from build123d import *

# Parameters (mm, degrees)
SKIZZE1_W                                            = 180
SKIZZE1_H                                            = 180
AUFSATZ_LINEAR_AUSTRAGEN1_DEPTH                      = 5
AUFSATZ_LINEAR_AUSTRAGEN2_DEPTH                      = 2
STIRNSENKUNG_F_R_M3_ZYLINDERSCHRAUBE_MIT_D           = 3.6
STIRNSENKUNG_F_R_M3_ZYLINDERSCHRAUBE_MIT_DEPTH       = 9.1
STIRNSENKUNG_F_R_M3_ZYLINDERSCHRAUBE_MIT_CBORE_D     = 6.5
STIRNSENKUNG_F_R_M3_ZYLINDERSCHRAUBE_MIT_CBORE_DEPTH = 3.4
STIRNSENKUNG_F_R_M3_ZYLINDERSCHRAUBE_MIT_TIP         = 1.081549114
VERRUNDUNG1_R                                        = 10
VERRUNDUNG2_R                                        = 2


with BuildPart() as part:
    # Skizze1 → Aufsatz-Linear austragen1 (new body)
    with BuildSketch(Plane(origin=(0, 0, 0), x_dir=(1, 0, 0), z_dir=(0, 1, 0))):
        Rectangle(SKIZZE1_W, SKIZZE1_H)
    extrude(amount=AUFSATZ_LINEAR_AUSTRAGEN1_DEPTH)

    # Skizze2 → Aufsatz-Linear austragen2 (add)
    with BuildSketch(Plane(origin=(0, 5, 0), x_dir=(1, 0, 0), z_dir=(0, 1, 0))):
        with BuildLine():
            Line((78, 85), (-78, 85))
            ThreePointArc((-78, 85), (-85.071067812, 82.071067812), (-88, 75))
            Line((-88, 75), (-88, -75))
            ThreePointArc((-88, -75), (-85.071067812, -82.071067812), (-78, -85))
            Line((-78, -85), (78, -85))
            ThreePointArc((78, -85), (85.071067812, -82.071067812), (88, -75))
            Line((88, -75), (88, 75))
            ThreePointArc((88, 75), (85.071067812, 82.071067812), (78, 85))
        make_face()
    extrude(amount=AUFSATZ_LINEAR_AUSTRAGEN2_DEPTH)

    # Stirnsenkung für M3 Zylinderschraube mit Innensechskant2
    with Locations(Plane(origin=(0, 0, 0), x_dir=(-1, 0, 0), z_dir=(0, -1, 0))):
        with Locations((-83, 80), (83, 80), (83, -80), (-83, -80)):
            CounterBoreHole(STIRNSENKUNG_F_R_M3_ZYLINDERSCHRAUBE_MIT_D / 2, STIRNSENKUNG_F_R_M3_ZYLINDERSCHRAUBE_MIT_CBORE_D / 2, STIRNSENKUNG_F_R_M3_ZYLINDERSCHRAUBE_MIT_CBORE_DEPTH, depth=STIRNSENKUNG_F_R_M3_ZYLINDERSCHRAUBE_MIT_DEPTH)
            with Locations((0, 0, -(STIRNSENKUNG_F_R_M3_ZYLINDERSCHRAUBE_MIT_DEPTH + STIRNSENKUNG_F_R_M3_ZYLINDERSCHRAUBE_MIT_TIP / 2))):  # 118° drill point
                Cone(0, STIRNSENKUNG_F_R_M3_ZYLINDERSCHRAUBE_MIT_D / 2, STIRNSENKUNG_F_R_M3_ZYLINDERSCHRAUBE_MIT_TIP, mode=Mode.SUBTRACT)

    # Verrundung1
    verrundung1_edges = [part.edges().sort_by_distance(p)[0] for p in [
        (90, 2.5, -90),
        (90, 2.5, 90),
        (-90, 2.5, 90),
        (-90, 2.5, -90),
    ]]
    fillet(verrundung1_edges, radius=VERRUNDUNG1_R)

    # Verrundung2
    verrundung2_edges = [part.edges().sort_by_distance(p)[0] for p in [
        (90, 0, 0),
        (0, 0, -90),
        (0, 0, 90),
        (-90, 0, 0),
        (87.071067812, 0, -87.071067812),
        (-87.071067812, 0, -87.071067812),
        (-87.071067812, 0, 87.071067812),
        (87.071067812, 0, 87.071067812),
    ]]
    fillet(verrundung2_edges, radius=VERRUNDUNG2_R)


solid = part.part
Could you check a few things on this model? Use its own coordinates, in mm. A direction names the side the tool comes from. Give positions to 0.01 mm unless a question says otherwise; leave off trailing zeros. Write each loop counter-clockwise with the first axis right and the second up, starting at its lowest first coordinate (ties: lowest second). Pieces come first, ordered by that corner, then holes. Notation, with made-up numbers: (79.25, 34.25) - (105.25, 34.25) arc R18 ccw to (105.25, 64.25) - close; hole circle Ø7 at (-22, -7). An arc over 180 degrees is marked (long way). Use CSV: the item, a comma, the result in double quotes. Start each with the question number.
Item 1: For faces 1 (the face through (-85.15, 5.99, 81.99)), 2 (the face through (-84.4, 3.4, 81.4)), 3 (the face through (84.99, 5.99, 82.15)), 4 (the face through (-84.99, 5.99, -82.15)), which set-ups out of +Z, -Z, +X, -X, +Y, -Y let a thin tool reach every point of the face, with its end or its side?
Item 2: I'm going to push flat-ended pins straight in: pin 1 (4 mm diameter, centred on x = -83, z = 80, fed in from -Y); pin 2 (1 mm diameter, centred on y = 6, z = 16.5, fed in from -X); pin 3 (1.6 mm diameter, centred on x = 9.5, y = 6, fed in from -Z). Where does each tip first touch, or does it pass through?
Item 3: I want a section at A-A, the plane x = -65. Please give me the cut outline in (y, z).
Item 4: If I drill on line 1 along X through (y, z) = (2.75, 77); line 2 along X through (y, z) = (1.4, 80); line 3 along Z through (x, y) = (83, 1.75), over which ranges is the centre line in solid material (lowest first)?
Item 5: If we mould it in two halves opening along Z, with no side actions, what happens to faces 5 (the face through (-80.421, 1.676, 81.978)), 6 (the face through (-1, 7, -1)), 7 (the face through (-87.15, 3.52, -86.99))? For each: pulls with the +Z half, pulls with the -Z half, needs draft (parallel to the pull), parting line crosses it, or undercut.
Findings:
1,face 1,"+Z, -X, +Y"
1,face 2,"-Y"
1,face 3,"+Z, +X, +Y"
1,face 4,"-Z, -X, +Y"
2,pin 1,"stops at y = 3.4"
2,pin 2,"stops at x = -88"
2,pin 3,"stops at z = -85"
3,outline,"(0, -88) arc R2 ccw to (2, -90) - (5, -90) - (5, -85) - (7, -85) - (7, 85) - (5, 85) - (5, 90) - (2, 90) arc R2 ccw to (0, 88) - close"
4,line 1,"x = -90 to -84.25, -81.75 to 81.75, 84.25 to 90"
4,line 2,"x = -89.91 to -86.25, -79.75 to 79.75, 86.25 to 89.91"
4,line 3,"z = -89.52 to -83.25, -76.75 to 76.75, 83.25 to 89.52"
5,face 5,"undercut"
5,face 6,"needs draft"
5,face 7,"pulls with the -Z half"
